Here's how the part is built. I have some questions about the finished solid (model axes, mm). A direction names the side the tool comes from. Round coordinates to 2 decimals unless told otherwise and drop trailing zeros. Write each loop counter-clockwise with the first axis right and the second up, starting at its lowest first coordinate (ties: lowest second). Pieces come first, ordered by that corner, then holes. Notation, with made-up numbers: (7, 16) -> (64, 16) arc R35 cw to (64, 52) -> close; hole circle Ø4 at (-5, 2). An arc over 180 degrees is marked (long way). Answer in a Markdown table with one row per item.
from build123d import *

# Parameters (mm, degrees)
SKETCH1_R                = 11
SKETCH1_R_2              = 1.5
BOSS_EXTRUDE1_DEPTH      = 2
BOSS_EXTRUDE2_DEPTH      = 20
BOSS_EXTRUDE2_DEPTH_BACK = 2
SKETCH2_W                = 50
SKETCH2_H                = 2


with BuildPart() as part:
    # Sketch1 → Boss-Extrude1 (new body)
    with BuildSketch(Plane.XY):
        with BuildLine():
            Line((-25, -20), (25, -20))
            Line((25, -20), (17.201468929, 5.301836161))
            ThreePointArc((17.201468929, 5.301836161), (0, 18), (-17.201468929, 5.301836161))
            Line((-17.201468929, 5.301836161), (-25, -20))
        make_face()
        Circle(SKETCH1_R, mode=Mode.SUBTRACT)
        with Locations((0, 14)):
            Circle(SKETCH1_R_2, mode=Mode.SUBTRACT)
        with Locations((14, 0)):
            Circle(SKETCH1_R_2, mode=Mode.SUBTRACT)
        with Locations((0, -14)):
            Circle(SKETCH1_R_2, mode=Mode.SUBTRACT)
        with Locations((-14, 0)):
            Circle(SKETCH1_R_2, mode=Mode.SUBTRACT)
    extrude(amount=BOSS_EXTRUDE1_DEPTH)

    # Sketch2 → Boss-Extrude2 (add, two sides: drawn at the far end of the back side and taken through both)
    with BuildSketch(Plane.XY.offset(2).offset(-BOSS_EXTRUDE2_DEPTH_BACK)):
        with Locations((0, -21)):
            Rectangle(SKETCH2_W, SKETCH2_H)
    extrude(amount=BOSS_EXTRUDE2_DEPTH + BOSS_EXTRUDE2_DEPTH_BACK)


solid = part.part
1) For pin 1 (12 mm diameter, centred on y = 0, z = 4.5, fed in from -X); pin 2 (5 mm diameter, centred on x = 0, y = -14, fed in from +Z), each with a flat end and sliding along its axis, tell me the tip position at first contact or that it passes through.
Response:
| item | result |
|---|---|
| pin 1 | stops at x = -20.52 |
| pin 2 | stops at z = 2 |
2) I want a section at A-A, the plane y = 14. List the corners of the cut face in (x, z) for me.
Response:
| item | result |
|---|---|
| outline | (-11.31, 0) -> (-1.5, 0) -> (-1.5, 2) -> (-11.31, 2) -> close; (1.5, 0) -> (11.31, 0) -> (11.31, 2) -> (1.5, 2) -> close |
3) We'd pull the mould along Y, two halves only. Please class faces 1 (the face through (0, 18, 1)), 2 (the face through (-0.325, -15.464, 0.986)), 3 (the face through (-25, -21, 11)): +Y half, -Y half, draft (parallel to the pull), parting line (faces both ways), or undercut.
Response:
| item | result |
|---|---|
| face 1 | +Y half |
| face 2 | undercut |
| face 3 | draft |
4) I want a section at B-B, the plane x = -6.5. List the corners of the cut face in (y, z) for me, and give its area (3 significant figures).
Response:
| item | result |
|---|---|
| outline | (-22, 0) -> (-8.87, 0) -> (-8.87, 2) -> (-20, 2) -> (-20, 22) -> (-22, 22) -> close; (8.87, 0) -> (16.79, 0) -> (16.79, 2) -> (8.87, 2) -> close |
| area | 82.1 mm^2 |
5) Which directions (+Z, -Z, +X, -X, +Y, -Y) give clear straight access to the entire face, cutting with the end or side of a thin tool? Please do faces 4 (the face through (12.5, 0.07, 0.99)), 5 (the face through (0, -20, 12)).
Response:
| item | result |
|---|---|
| face 4 | +Z, -Z |
| face 5 | +Z, +X, -X, +Y |
6) I want a section at C-C, the plane y = 0. List the corners of the cut face in (x, z) for me.
Response:
| item | result |
|---|---|
| outline | (-18.84, 0) -> (-15.5, 0) -> (-15.5, 2) -> (-18.84, 2) -> close; (-12.5, 0) -> (-11, 0) -> (-11, 2) -> (-12.5, 2) -> close; (11, 0) -> (12.5, 0) -> (12.5, 2) -> (11, 2) -> close; (15.5, 0) -> (18.84, 0) -> (18.84, 2) -> (15.5, 2) -> close |
7) I want a section at D-D, the plane z = 18.75. List the corners of the cut face in (x, y) for me, and give its area (3 significant figures).
Response:
| item | result |
|---|---|
| outline | (-25, -22) -> (25, -22) -> (25, -20) -> (-25, -20) -> close |
| area | 100 mm^2 |
8) I need wall thicknesses on line 1 (Y direction, x = 0, z = 0.7); line 2 (Y direction, x = 10, z = 21); line 3 (Z direction, x = -12.5, y = -19). Which ranges of each line are inside material? Lowest first, please. Write a range as [from, to].
Response:
| item | result |
|---|---|
| line 1 | y = [-22, -15.5], [-12.5, -11], [11, 12.5], [15.5, 18] |
| line 2 | y = [-22, -20] |
| line 3 | z = [0, 2] |
